Build history of the part. All positions in model axes, mm. A direction names the side the tool comes from. Round coordinates to 2 decimals unless told otherwise and drop trailing zeros. Loops run counter-clockwise (first coordinate to the right, second up) from the corner with the lowest first, then second, coordinate; pieces in that order, holes last.
from build123d import *

# Parameters (mm, degrees)
SKETCH1_W               = 66
SKETCH1_H               = 66
BOSS_EXTRUDE1_DEPTH     = 40
SKETCH2_R               = 25
CUT_EXTRUDE1_DEPTH      = 31
SKETCH3_R               = 6.25
CUT_EXTRUDE2_DEPTH      = 7
SKETCH4_W               = 12.5
SKETCH4_H               = 31
CUT_EXTRUDE3_DEPTH      = 1
CUT_EXTRUDE3_DEPTH_BACK = 67
SKETCH5_R               = 2
CUT_EXTRUDE4_DEPTH      = 10


with BuildPart() as part:
    # Sketch1 → Boss-Extrude1 (new body)
    with BuildSketch(Plane(origin=(0, 0, 0), x_dir=(1, 0, 0), z_dir=(0, 1, 0))):
        Rectangle(SKETCH1_W, SKETCH1_H)
    extrude(amount=BOSS_EXTRUDE1_DEPTH)

    # Sketch2 → Cut-Extrude1 (cut)
    with BuildSketch(Plane(origin=(0, 40, 0), x_dir=(1, 0, 0), z_dir=(0, 1, 0))):
        Circle(SKETCH2_R)
    extrude(amount=-CUT_EXTRUDE1_DEPTH, mode=Mode.SUBTRACT)

    # Sketch3 → Cut-Extrude2 (cut)
    with BuildSketch(Plane(origin=(0, 9, 0), x_dir=(1, 0, 0), z_dir=(0, 1, 0))):
        Circle(SKETCH3_R)
    extrude(amount=-CUT_EXTRUDE2_DEPTH, mode=Mode.SUBTRACT)

    # Sketch4 → Cut-Extrude3 (cut, two sides)
    with BuildSketch(Plane.XY.offset(33)) as cut_extrude3_sk:
        with Locations((18.75, 24.5)):
            Rectangle(SKETCH4_W, SKETCH4_H)
    extrude(amount=CUT_EXTRUDE3_DEPTH, mode=Mode.SUBTRACT)
    extrude(cut_extrude3_sk.sketch, amount=-CUT_EXTRUDE3_DEPTH_BACK, mode=Mode.SUBTRACT)

    # Sketch5 → Cut-Extrude4 (cut)
    with BuildSketch(Plane(origin=(0, 40, 0), x_dir=(1, 0, 0), z_dir=(0, 1, 0))):
        with Locations((-29, -29)):
            Circle(SKETCH5_R)
        with Locations((-29, 29)):
            Circle(SKETCH5_R)
        with Locations((29, 29)):
            Circle(SKETCH5_R)
        with Locations((29, -29)):
            Circle(SKETCH5_R)
    extrude(amount=-CUT_EXTRUDE4_DEPTH, mode=Mode.SUBTRACT)


solid = part.part
(1) Slice it at A-A on y = 10. List the corners of the cut face in (x, z), plus the area to 3 significant figures.
Responses:
outline: (-33, -33) - (12.5, -33) - (12.5, -21.65) arc R25 cw (long way) to (12.5, 21.65) - (12.5, 33) - (-33, 33) - close; (25, -33) - (33, -33) - (33, 33) - (25, 33) - close
area: 1,950 mm2
(2) Pull direction Z, two halves, no side cores. Call faces 4 (the face through (29, 40, 0)), 5 (the face through (-8, 20, 33)), 6 (the face through (-24.99, 24.72, -0.73)), 7 (the face through (0, 2, 0)): +Z half, -Z half, draft (parallel to the pull), parting line (faces both ways), or undercut.
Responses:
face 4: draft
face 5: +Z half
face 6: undercut
face 7: undercut
(3) Slice it at D-D on y = 4. List the corners of the cut face in (x, z), plus the area to 3 significant figures.
Responses:
outline: (-33, -33) - (33, -33) - (33, 33) - (-33, 33) - close; hole circle Ø12.5 at (0, 0)
area: 4,230 mm2
(4) Probe line 1 (X direction, y = 33, z = 29); line 2 (Z direction, x = 29, y = 36); line 3 (X direction, y = 5.75, z = 0). List the from-to ranges inside material, lowest first.
Responses:
line 1: x = -33 to -31, -27 to 12.5, 25 to 27, 31 to 33
line 2: z = -33 to -31, -27 to 27, 31 to 33
line 3: x = -33 to -6.25, 6.25 to 33
(5) Slice it at B-B on z = -29. List the corners of the cut face in (x, y), plus the area to 3 significant figures.
Responses:
outline: (-33, 0) - (33, 0) - (33, 40) - (31, 40) - (31, 30) - (27, 30) - (27, 40) - (25, 40) - (25, 9) - (12.5, 9) - (12.5, 40) - (-27, 40) - (-27, 30) - (-31, 30) - (-31, 40) - (-33, 40) - close
area: 2,170 mm2
(6) Which spindle directions (+Z, -Z, +X, -X, +Y, -Y) get a long thin tool onto all of the face, cutting with end or side? Do faces 1 (the face through (25, 24, 0)), 2 (the face through (29, 30, -29)), 3 (the face through (-26, 40, 0)). Say none if no direction does.
Responses:
face 1: +Z, -Z, +Y
face 2: +Y
face 3: +Z, -Z, +X, -X, +Y
(7) Slice it at C-C on x = 29. List the corners of the cut face in (y, z), plus the area to 3 significant figures.
Responses:
outline: (0, -33) - (40, -33) - (40, -31) - (30, -31) - (30, -27) - (40, -27) - (40, 27) - (30, 27) - (30, 31) - (40, 31) - (40, 33) - (0, 33) - close
area: 2,560 mm2
(8) Pin check, flat tips, straight feed: P1, Ø10, axis at x = 0, z = 0, coming from the +Y side; P2, Ø1.2, axis at x = -29.5, z = 29, coming from the +Y side; P3, Ø4, axis at x = 2.5, z = 12, coming from the +Y side. Stop position of each tip, or through.
Responses:
P1: stops at y = 2
P2: stops at y = 30
P3: stops at y = 9
